Answer from the drawing. Dimensions are ordinates in mm from the lowest x, y and z of the part. A direction names the side the tool comes from. Give positions to 0.01 mm unless a question says otherwise; leave off trailing zeros. Order: outer loops, then holes, each group sorted by start corner. A loop starts at its lowest first (then second) coordinate and runs counter-clockwise, first axis right, second up. Notation, with made-up numbers: (36.5, -13.5) - (78.5, -13.5) arc R34 cw to (78.5, 25.5) - close; hole circle Ø10 at (68.5, 79). An arc over 180 degrees is marked (long way). One line per item, written item: value. Start each with the question number.
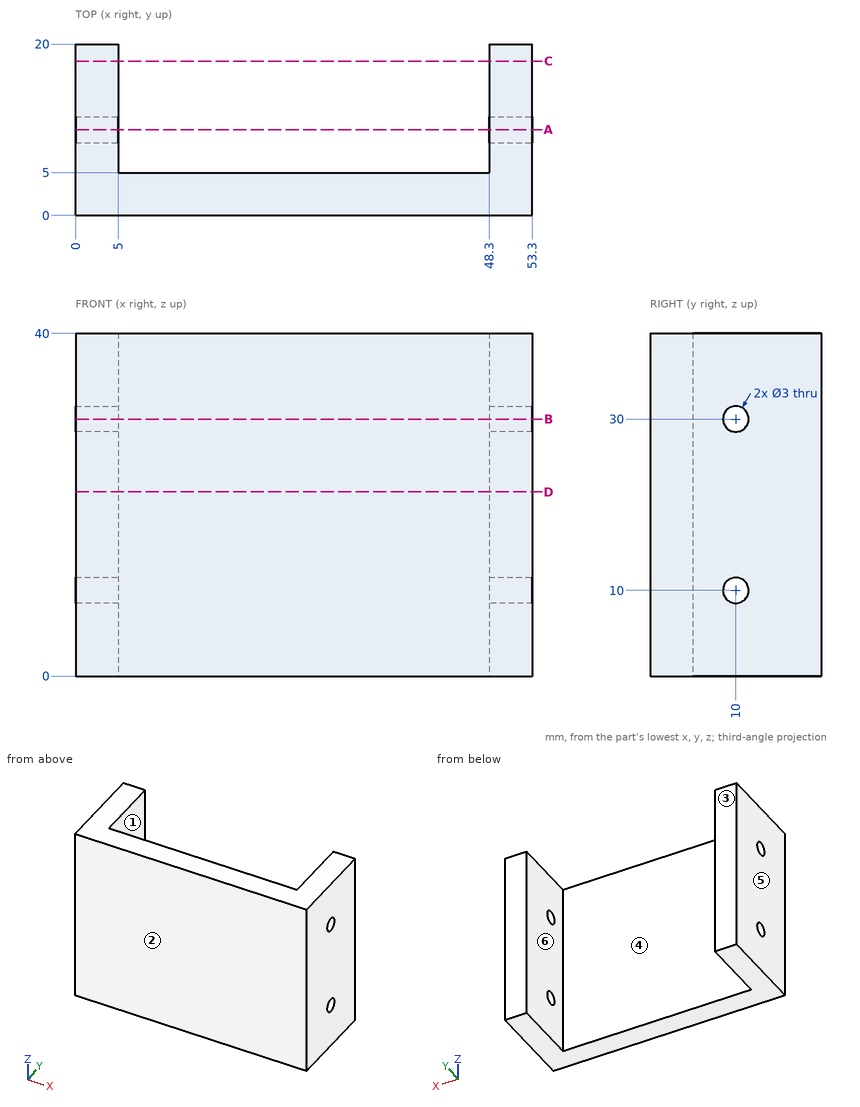
1) Section A-A on y = 10 is taken. Write down the section's boundary in (x, z), plus the area to 3 significant figures.
2) Section C-C on y = 18 is taken. Write down the section's boundary in (x, z).
3) Section D-D on z = 21.5 is taken. Write down the section's boundary in (x, y), plus the area to 4 significant figures.
4) Find the intervals of material crossed by probe 1 along Y at (x, z) = (1.5, 10); probe 2 along X at (y, z) = (8.25, 22.5); probe 3 along Y at (x, z) = (36.5, 33.5), in increasing order. Write a range as from..to.
5) Section B-B on z = 30 is taken. Write down the section's boundary in (x, y), plus the area to 4 significant figures.
6) For the marked faces 1 and 2, determine the directions among +Z, -Z, +X, -X, +Y, -Y from which every point of the face is accessible in a straight line to the end or side of a thin tool.
7) Each of these flat-tipped pins is pushed along its axis until it touches: pin 1 (1.5 mm diameter, centred on x = 31.5, z = 33.5, fed in from +Y); pin 2 (2.5 mm diameter, centred on y = 10, z = 30, fed in from -X); pin 3 (5 mm diameter, centred on y = 10, z = 10, fed in from -X). Where does it stop, or does it pass through?
8) The mould has two halves that part along X. Classify the marked faces 3, 4, 5 and 6: +X half, -X half, draft (parallel to the pull), parting line (faces both ways), or undercut.
Solved:
1. outline: (0, 0) - (5, 0) - (5, 8.5) - (0, 8.5) - close; (0, 11.5) - (5, 11.5) - (5, 28.5) - (0, 28.5) - close; (0, 31.5) - (5, 31.5) - (5, 40) - (0, 40) - close; (48.3, 0) - (53.3, 0) - (53.3, 8.5) - (48.3, 8.5) - close; (48.3, 11.5) - (53.3, 11.5) - (53.3, 28.5) - (48.3, 28.5) - close; (48.3, 31.5) - (53.3, 31.5) - (53.3, 40) - (48.3, 40) - close
1. area: 340 mm2
2. outline: (0, 0) - (5, 0) - (5, 40) - (0, 40) - close; (48.3, 0) - (53.3, 0) - (53.3, 40) - (48.3, 40) - close
3. outline: (0, 0) - (53.3, 0) - (53.3, 20) - (48.3, 20) - (48.3, 5) - (5, 5) - (5, 20) - (0, 20) - close
3. area: 416.5 mm2
4. probe 1: y = 0..8.5, 11.5..20
4. probe 2: x = 0..5, 48.3..53.3
4. probe 3: y = 0..5
5. outline: (0, 0) - (53.3, 0) - (53.3, 8.5) - (48.3, 8.5) - (48.3, 5) - (5, 5) - (5, 8.5) - (0, 8.5) - close; (0, 11.5) - (5, 11.5) - (5, 20) - (0, 20) - close; (48.3, 11.5) - (53.3, 11.5) - (53.3, 20) - (48.3, 20) - close
5. area: 386.5 mm2
6. face 1: +Z, -Z, +Y
6. face 2: +Z, -Z, +X, -X, -Y
7. pin 1: stops at y = 5
7. pin 2: passes through
7. pin 3: stops at x = 0
8. face 3: draft
8. face 4: undercut
8. face 5: -X half
8. face 6: undercut
